from build123d import *

# Parameters (mm, degrees)
SKETCH2_W           = 273.05
SKETCH2_H           = 273.05
SKETCH2_R           = 2.54
BOSS_EXTRUDE1_DEPTH = 6.35
SKETCH3_W           = 60.96
SKETCH3_H           = 17.280059867
CUT_EXTRUDE1_DEPTH  = 194.179899964


with BuildPart() as part:
    # Sketch2 → Boss-Extrude1 (new body)
    with BuildSketch(Plane.XY):
        Rectangle(SKETCH2_W, SKETCH2_H)
        with Locations((-120.396, 123.825)):
            Circle(SKETCH2_R, mode=Mode.SUBTRACT)
        with Locations((-120.396, 73.787)):
            Circle(SKETCH2_R, mode=Mode.SUBTRACT)
        with Locations((0, 123.825)):
            Circle(SKETCH2_R, mode=Mode.SUBTRACT)
        with Locations(Location((120.396, 73.787, 0), (0, 0, 180))):
            Circle(SKETCH2_R, mode=Mode.SUBTRACT)
        with Locations(Location((120.396, 123.825, 0), (0, 0, 180))):
            Circle(SKETCH2_R, mode=Mode.SUBTRACT)
        with Locations((120.396, -123.825)):
            Circle(SKETCH2_R, mode=Mode.SUBTRACT)
        with Locations((120.396, -73.787)):
            Circle(SKETCH2_R, mode=Mode.SUBTRACT)
        with Locations(Location((0, -123.825, 0), (0, 0, 180))):
            Circle(SKETCH2_R, mode=Mode.SUBTRACT)
        with Locations(Location((-120.396, -73.787, 0), (0, 0, 180))):
            Circle(SKETCH2_R, mode=Mode.SUBTRACT)
        with Locations(Location((-120.396, -123.825, 0), (0, 0, 180))):
            Circle(SKETCH2_R, mode=Mode.SUBTRACT)
    extrude(amount=BOSS_EXTRUDE1_DEPTH)

    # Sketch3 → Cut-Extrude1 (cut, through all)
    with BuildSketch(Plane.XY.offset(6.35)):
        with Locations((73.66, 137.545029934)):
            Rectangle(SKETCH3_W, SKETCH3_H)
        with Locations((-73.66, 137.545029934)):
            Rectangle(SKETCH3_W, SKETCH3_H)
        with Locations((-73.66, -137.545029934)):
            Rectangle(SKETCH3_W, SKETCH3_H)
        with Locations((73.66, -137.545029934)):
            Rectangle(SKETCH3_W, SKETCH3_H)
    extrude(amount=-CUT_EXTRUDE1_DEPTH, mode=Mode.SUBTRACT)


solid = part.part
Model file for the job. Use its own axes, mm. A direction names the side the tool comes from. Give positions to 0.01 mm unless a question says otherwise; leave off trailing zeros. Loops run counter-clockwise (first coordinate to the right, second up) from the corner with the lowest first, then second, coordinate; pieces in that order, holes last.
1) Flat gauge pins, fed straight in: pin 1 Ø3 at (x, z) = (-86, 3) entering from -Y (3 decimals); pin 2 Ø4 at (x, y) = (-7, 103) entering from -Z; pin 3 Ø3 at (x, y) = (-120.396, -73.787) entering from +Z. Where does each tip first touch, or does it go through?
2) Tool access for faces 4 (the flat face through (-1, 136.525, 3)), 5 (the flat face through (-74, -128.905, 3)), 6 (the flat face through (-74, 128.905, 3)): list every direction of +Z, -Z, +X, -X, +Y, -Y with a clear straight run to the whole face (end or side of a thin tool).
3) Saw through at A-A (z = 2.75). Count the separate pieces of the cut face and the enclosed holes in it, plus the area to 3 significant figures.
4) Pull direction X, two halves, no side cores. Call faces 1 (the flat face through (-43.18, 133, 3)), 2 (the flat face through (136.525, -2, 3)), 3 (the flat face through (120, -136.525, 3)): +X half, -X half, draft (parallel to the pull), parting line (faces both ways), or undercut.
5) Saw through at B-B (x = -97). Write the cut outline in (y, z) (3 decimals), plus the area to 3 significant figures.
6) Wall check: line 1 (X direction, y = 75.5, z = 1.25) (3 decimals); line 2 (Y direction, x = -121.5, z = 4) (3 decimals); line 3 (X direction, y = -123, z = 2.5) (3 decimals). Give the ranges that are in metal, low to high.
Answer block:
1. pin 1: stops at y = -128.905
1. pin 2: stops at z = 0
1. pin 3: passes through
2. face 4: +Z, -Z, +X, -X, +Y
2. face 5: +Z, -Z, -Y
2. face 6: +Z, -Z, +Y
3. separate pieces: 1
3. enclosed holes: 10
3. area: 72,500 mm2
4. face 1: undercut
4. face 2: +X half
4. face 3: draft
5. outline: (-128.905, 0) - (128.905, 0) - (128.905, 6.35) - (-128.905, 6.35) - close
5. area: 1,640 mm2
6. line 1: x = -136.525 to -122.271, -118.521 to 118.521, 122.271 to 136.525
6. line 2: y = -136.525 to -126.113, -121.537 to -76.075, -71.499 to 71.499, 76.075 to 121.537, 126.113 to 136.525
6. line 3: x = -136.525 to -122.798, -117.994 to -2.402, 2.402 to 117.994, 122.798 to 136.525
